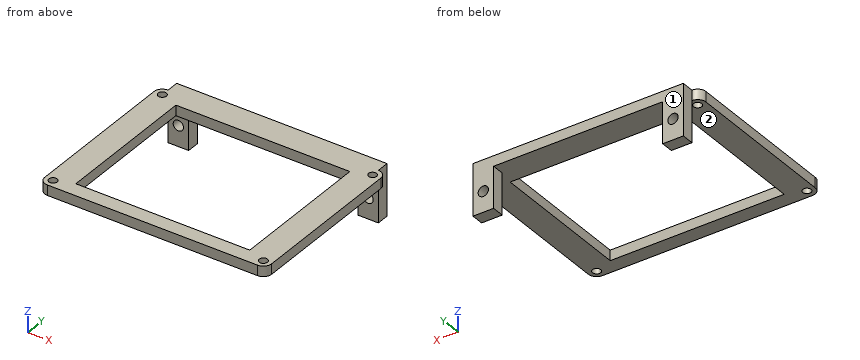
```python
from build123d import *

# Parameters (mm, degrees)
SKETCH_1_R          = 1.945914192
SKETCH_1_R_2        = 2
EXTRUDE_1_DEPTH     = 5
SKETCH_2_W          = 10
SKETCH_2_H          = 20
SKETCH_2_R          = 2.5
SKETCH_2_H_2        = 5
SKETCH_2_W_2        = 82
EXTRUDE_2_DEPTH     = 6
SKETCH_3_W          = 84.346489647
SKETCH_3_H          = 69.622064444
CUT_EXTRUDE_1_DEPTH = 6


with BuildPart() as part:
    # 草图1 → 凸台-拉伸1 (new body)
    with BuildSketch(Plane.XY):
        with BuildLine():
            Line((-34.088642659, 27.271468144), (67.911357341, 27.271468144))
            ThreePointArc((67.911357341, 27.271468144), (70.739784465, 26.099895269), (71.911357341, 23.271468144))
            Line((71.911357341, 23.271468144), (71.911357341, -52.728531856))
            ThreePointArc((71.911357341, -52.728531856), (70.739784465, -55.556958981), (67.911357341, -56.728531856))
            Line((67.911357341, -56.728531856), (-34.088642659, -56.728531856))
            ThreePointArc((-34.088642659, -56.728531856), (-36.917069784, -55.556958981), (-38.088642659, -52.728531856))
            Line((-38.088642659, -52.728531856), (-38.088642659, 23.271468144))
            ThreePointArc((-38.088642659, 23.271468144), (-36.917069784, 26.099895269), (-34.088642659, 27.271468144))
        make_face()
        with Locations((67.911357341, 23.271468144)):
            Circle(SKETCH_1_R, mode=Mode.SUBTRACT)
        with Locations((-34.088642659, 23.271468144)):
            Circle(SKETCH_1_R_2, mode=Mode.SUBTRACT)
        with Locations((67.911357341, -52.728531856)):
            Circle(SKETCH_1_R_2, mode=Mode.SUBTRACT)
        with Locations((-34.088642659, -52.728531856)):
            Circle(SKETCH_1_R_2, mode=Mode.SUBTRACT)
    extrude(amount=EXTRUDE_1_DEPTH)

    # 草图2 → 凸台-拉伸2 (add)
    # profile 1 of 5: a face of its own
    with BuildSketch(Plane(origin=(0, 27.271468144, 0), x_dir=(1, 0, 0), z_dir=(0, 1, 0))):
        with Locations((-29.088642659, 10)):
            Rectangle(SKETCH_2_W, SKETCH_2_H)
        with Locations(Location((-29.088642659, 10, 0), (0, 0, 270))):
            Circle(SKETCH_2_R, mode=Mode.SUBTRACT)
    # profile 2 of 5: a face of its own
    with BuildSketch(Plane(origin=(0, 27.271468144, 0), x_dir=(1, 0, 0), z_dir=(0, 1, 0))):
        with Locations((-29.088642659, -2.5)):
            Rectangle(SKETCH_2_W, SKETCH_2_H_2)
    # profile 3 of 5: a face of its own
    with BuildSketch(Plane(origin=(0, 27.271468144, 0), x_dir=(1, 0, 0), z_dir=(0, 1, 0))):
        with Locations((16.911357341, -2.5)):
            Rectangle(SKETCH_2_W_2, SKETCH_2_H_2)
    # profile 4 of 5: a face of its own
    with BuildSketch(Plane(origin=(0, 27.271468144, 0), x_dir=(1, 0, 0), z_dir=(0, 1, 0))):
        with Locations((62.911357341, 10)):
            Rectangle(SKETCH_2_W, SKETCH_2_H)
        with Locations(Location((62.911357341, 10, 0), (0, 0, 270))):
            Circle(SKETCH_2_R, mode=Mode.SUBTRACT)
    # profile 5 of 5: a face of its own
    with BuildSketch(Plane(origin=(0, 27.271468144, 0), x_dir=(1, 0, 0), z_dir=(0, 1, 0))):
        with Locations((62.911357341, -2.5)):
            Rectangle(SKETCH_2_W, SKETCH_2_H_2)
    extrude(amount=EXTRUDE_2_DEPTH)

    # 草图3 → 切除-拉伸1 (cut)
    with BuildSketch(Plane.XY.offset(5)):
        with Locations((16.911357341, -14.728531856)):
            Rectangle(SKETCH_3_W, SKETCH_3_H)
    extrude(amount=-CUT_EXTRUDE_1_DEPTH, mode=Mode.SUBTRACT)


solid = part.part
```
Input: part model. Units: mm. Frame: model coordinates. Face numbers are marked on the shaded views. Coordinates: 2 decimals unless noted, no trailing zeros. Write each loop counter-clockwise with the first axis right and the second up, starting at its lowest first coordinate (ties: lowest second). Pieces come first, ordered by that corner, then holes. Notation, with made-up numbers: (38, -1) -> (59, -1) arc R26 ccw to (59, 27) -> close; hole circle Ø1 at (67, -26.5). An arc over 180 degrees is marked (long way). Write each question's results on one line, items separated by ' | '.
Item 1: Material intervals for probe 1 along X at (y, z) = (29.1, -10); probe 2 along Y at (x, z) = (-11.5, 3.75); probe 3 along X at (y, z) = (15, 1.5), sorted ascending.
Conclusion:
probe 1: x = -34.09 to -31.59, -26.59 to -24.09, 57.91 to 60.41, 65.41 to 67.91 | probe 2: y = -56.73 to -49.54, 20.08 to 33.27 | probe 3: x = -38.09 to -25.26, 59.08 to 71.91
Item 2: Section query C-C on y = 8. Return loops of the section in (x, z), plus the area to 3 significant figures.
Conclusion:
outline: (-38.09, 0) -> (-25.26, 0) -> (-25.26, 5) -> (-38.09, 5) -> close; (59.08, 0) -> (71.91, 0) -> (71.91, 5) -> (59.08, 5) -> close | area: 128 mm^2
Item 3: Section query B-B on x = 39. Return loops of the section in (y, z).
Conclusion:
outline: (-56.73, 0) -> (-49.54, 0) -> (-49.54, 5) -> (-56.73, 5) -> close; (20.08, 0) -> (33.27, 0) -> (33.27, 5) -> (20.08, 5) -> close
Item 4: Section query A-A on z = -10. Return loops of the section in (x, y), plus the area to 3 significant figures.
Conclusion:
outline: (-34.09, 27.27) -> (-31.59, 27.27) -> (-31.59, 33.27) -> (-34.09, 33.27) -> close; (-26.59, 27.27) -> (-24.09, 27.27) -> (-24.09, 33.27) -> (-26.59, 33.27) -> close; (57.91, 27.27) -> (60.41, 27.27) -> (60.41, 33.27) -> (57.91, 33.27) -> close; (65.41, 27.27) -> (67.91, 27.27) -> (67.91, 33.27) -> (65.41, 33.27) -> close | area: 60.0 mm^2
Item 5: Mould query, pull axis X, two halves, no side actions, for the marked faces 1 and 2. Classes: +X half, -X half, draft (parallel to the pull), parting line (faces both ways), or undercut.
Conclusion:
face 1: draft | face 2: undercut
Item 6: Pin query (flat end, axial travel): pin 1 Ø5 at (y, z) = (31, -7.5) entering from -X; pin 2 Ø5 at (y, z) = (29.5, -9.5) entering from +X; pin 3 Ø5 at (x, y) = (-34.09, -52.73) entering from -Z. Return the tip coordinate at first contact, or that it passes through.
Conclusion:
pin 1: stops at x = -34.09 | pin 2: stops at x = 67.91 | pin 3: stops at z = 0
